from build123d import *

# Parameters (mm, degrees)
F0_W     = 203.2
F0_H     = 127
F1_DEPTH = 6.35
F2_W     = 3.175
F2_H     = 3.175
F3_DEPTH = 203.2
F4_W     = 3.175
F4_H     = 3.175
F5_DEPTH = 136.525


with BuildPart() as f1:
    # F0 (on Front) → F1 (new body)
    with BuildSketch(Plane.XZ):
        Rectangle(F0_W, F0_H)
    extrude(amount=F1_DEPTH)

    # F2 (on face) → F3 (join)
    with BuildSketch(Plane.YZ.offset(101.6)):
        Polygon((-3.175, 63.5), (0, 63.5), (0, 69.85), (-6.35, 69.85), (-6.35, 66.675), (-3.175, 66.675), align=None)
        with Locations((-1.5875, -65.0875)):
            Rectangle(F2_W, F2_H)
    extrude(amount=-F3_DEPTH)

    # F4 (on face) → F5 (join)
    with BuildSketch(Plane(origin=(0, 0, -66.675), x_dir=(1, 0, 0), z_dir=(0, 0, -1))):
        with Locations((-103.1875, 1.5875)):
            Rectangle(F4_W, F4_H)
        with Locations((103.1875, 1.5875)):
            Rectangle(F4_W, F4_H)
    extrude(amount=-F5_DEPTH)


solid = f1.part
Source: CAD feature listing. Evaluate the final solid. Frame: model axes, mm. Give positions to 0.01 mm unless a question says otherwise; leave off trailing zeros. Write each loop counter-clockwise with the first axis right and the second up, starting at its lowest first coordinate (ties: lowest second). Pieces come first, ordered by that corner, then holes. Notation, with made-up numbers: M -40,-4.75 L 13,-4.75 A18 cw 13,4.25 Z; hole C 46.5,-14.75 d6. An arc over 180 degrees is marked long. Return JSON: item names as keys, results as strings. Group by question number.
1) Cut plane B-B, the plane x = 5.5. Output: boundary loops of the cut face in (y, z) (3 decimals), plus the area to 3 significant figures.
2) Material intervals for line 1 along Z through (x, y) = (73, -4.75) (3 decimals); line 2 along X through (y, z) = (-4, -57.5), sorted ascending. Write a range as [from, to].
3) Pin query (flat end, axial travel): P1, Ø2, axis at y = -5, z = 52.5, coming from the +X side; P2, Ø1.6, axis at y = -4.5, z = -10.5, coming from the -X side; P3, Ø2.5, axis at x = 43, y = -5, coming from the -Z side. Return the tip coordinate at first contact, or that it passes through.
4) Cut plane C-C, the plane z = 31.5. Output: boundary loops of the cut face in (x, y) (3 decimals).
5) Cut plane A-A, the plane y = -5. Output: boundary loops of the cut face in (x, z) (3 decimals).
Recorded:
{
 "1": {"outline": "M -6.35,-63.5 L -3.175,-63.5 L -3.175,-66.675 L 0,-66.675 L 0,69.85 L -6.35,69.85 L -6.35,66.675 L -3.175,66.675 L -3.175,63.5 L -6.35,63.5 Z", "area": "847 mm²"},
 "2": {"line 1": "z = [-63.5, 63.5], [66.675, 69.85]", "line 2": "x = [-101.6, 101.6]"},
 "3": {"P1": "stops at x = 101.6", "P2": "stops at x = -101.6", "P3": "stops at z = -63.5"},
 "4": {"outline": "M -104.775,-3.175 L -101.6,-3.175 L -101.6,-6.35 L 101.6,-6.35 L 101.6,-3.175 L 104.775,-3.175 L 104.775,0 L -104.775,0 Z"},
 "5": {"outline": "M -101.6,-63.5 L 101.6,-63.5 L 101.6,63.5 L -101.6,63.5 Z; M -101.6,66.675 L 101.6,66.675 L 101.6,69.85 L -101.6,69.85 Z"}
}
